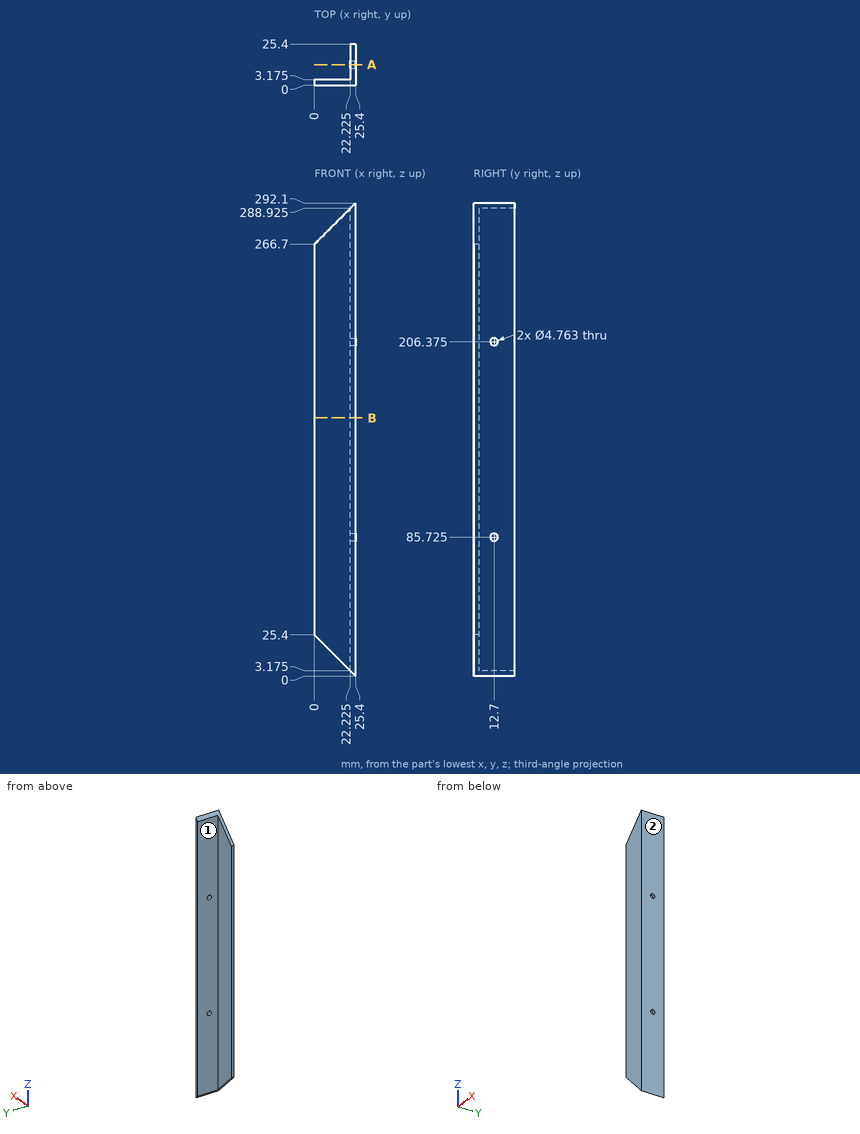
Can you work these out from the drawing? Everything is in mm from the part's minimum corner. A direction names the side the tool comes from. Coordinates: 2 decimals unless noted, no trailing zeros. Loops run counter-clockwise (first coordinate to the right, second up) from the corner with the lowest first, then second, coordinate; pieces in that order, holes last.
1. Imagine slicing it at A-A, the plane y = 12.7. Please give me the cut outline in (x, z) (1 decimal).
2. I need wall thicknesses on L1, parallel to Y at x = 10.5, z = 157 (1 decimal); L2, parallel to X at y = 13.5, z = 12.5 (1 decimal); L3, parallel to Z at x = 23.25, y = 21.75. Which ranges of each line are inside material? Lowest first, please.
3. For the marked faces 1 and 2, which set-ups out of +Z, -Z, +X, -X, +Y, -Y let a thin tool reach every point of the face, with its end or its side?
4. Imagine slicing it at B-B, the plane z = 159.5. Please give me the cut outline in (x, y) (1 decimal).
5. For P1, Ø2, axis at x = 3.5, y = 5, coming from the +Z side; P2, Ø2, axis at y = 15, z = 242.5, coming from the -X side (1 decimal); P3, Ø5, axis at x = 16.5, z = 103.5, coming from the +Y side (1 decimal); P4, Ø5.5, axis at y = 12.7, z = 85.725, coming from the +X side, each with a flat end and sliding along its axis, tell me the tip position at first contact or that it passes through.
Taken from the geometry:
1. outline: (22.2, 3.2) - (25.4, 0) - (25.4, 83.3) - (22.2, 83.3) - close; (22.2, 88.1) - (25.4, 88.1) - (25.4, 204) - (22.2, 204) - close; (22.2, 208.8) - (25.4, 208.8) - (25.4, 292.1) - (22.2, 288.9) - close
2. L1: y = 0 to 3.2
2. L2: x = 22.2 to 25.4
2. L3: z = 2.15 to 289.95
3. face 1: +Z, -Z, -X, +Y
3. face 2: +Z, -Z, +X, +Y, -Y
4. outline: (0, 0) - (25.4, 0) - (25.4, 25.4) - (22.2, 25.4) - (22.2, 3.2) - (0, 3.2) - close
5. P1: passes through
5. P2: stops at x = 22.2
5. P3: stops at y = 3.2
5. P4: stops at x = 25.4
